```python
from build123d import *

# Parameters (mm, degrees)
F0_R     = 42
F0_R_2   = 1.5
F1_DEPTH = 5
F2_R     = 2.49999
F3_SIZE  = 2


# Not quite as in the source:
# - a fillet or chamfer is up to 0.001 mm smaller than in the source, because OpenCascade refuses the exact size


with BuildPart() as f1:
    # F0 (on Top) → F1 (new body)
    with BuildSketch(Plane.XY):
        Circle(F0_R)
        with BuildLine():
            ThreePointArc((34.3681841493, 13.6144476452), (33.928844321, 12.5537874734), (32.8681841493, 12.1144476452))
            Line((32.8681841493, 12.1144476452), (32.8681841493, -12.1144476452))
            ThreePointArc((32.8681841493, -12.1144476452), (33.928844321, -12.5537874734), (34.3681841493, -13.6144476452))
            ThreePointArc((34.3681841493, -13.6144476452), (33.4422092978, -15.000266944), (31.8075239775, -14.675107817))
            Line((31.8075239775, -14.675107817), (14.675107817, -31.8075239775))
            ThreePointArc((14.675107817, -31.8075239775), (15.000266944, -32.2941590007), (15.1144476452, -32.8681841493))
            ThreePointArc((15.1144476452, -32.8681841493), (13.6144476452, -34.3681841493), (12.1144476452, -32.8681841493))
            Line((12.1144476452, -32.8681841493), (-12.1144476452, -32.8681841493))
            ThreePointArc((-12.1144476452, -32.8681841493), (-14.1884727937, -34.254003448), (-14.675107817, -31.8075239775))
            Line((-14.675107817, -31.8075239775), (-31.8075239775, -14.675107817))
            ThreePointArc((-31.8075239775, -14.675107817), (-34.254003448, -14.1884727937), (-32.8681841493, -12.1144476452))
            Line((-32.8681841493, -12.1144476452), (-32.8681841493, 12.1144476452))
            ThreePointArc((-32.8681841493, 12.1144476452), (-34.254003448, 14.1884727937), (-31.8075239775, 14.675107817))
            Line((-31.8075239775, 14.675107817), (-14.675107817, 31.8075239775))
            ThreePointArc((-14.675107817, 31.8075239775), (-14.1884727937, 34.254003448), (-12.1144476452, 32.8681841493))
            Line((-12.1144476452, 32.8681841493), (12.1144476452, 32.8681841493))
            ThreePointArc((12.1144476452, 32.8681841493), (13.6144476452, 34.3681841493), (15.1144476452, 32.8681841493))
            ThreePointArc((15.1144476452, 32.8681841493), (15.000266944, 32.2941590007), (14.675107817, 31.8075239775))
            Line((14.675107817, 31.8075239775), (31.8075239775, 14.675107817))
            ThreePointArc((31.8075239775, 14.675107817), (33.4422092978, 15.000266944), (34.3681841493, 13.6144476452))
        make_face(mode=Mode.SUBTRACT)
        with BuildLine():
            Line((32.8681841493, -12.1144476452), (32.8681841493, 12.1144476452))
            ThreePointArc((32.8681841493, 12.1144476452), (31.4823648505, 13.0404224967), (31.8075239775, 14.675107817))
            Line((31.8075239775, 14.675107817), (14.675107817, 31.8075239775))
            ThreePointArc((14.675107817, 31.8075239775), (13.0404224967, 31.4823648505), (12.1144476452, 32.8681841493))
            Line((12.1144476452, 32.8681841493), (-12.1144476452, 32.8681841493))
            ThreePointArc((-12.1144476452, 32.8681841493), (-13.0404224967, 31.4823648505), (-14.675107817, 31.8075239775))
            Line((-14.675107817, 31.8075239775), (-31.8075239775, 14.675107817))
            ThreePointArc((-31.8075239775, 14.675107817), (-31.4823648505, 14.1884727937), (-31.3681841493, 13.6144476452))
            ThreePointArc((-31.3681841493, 13.6144476452), (-31.8075239775, 12.5537874734), (-32.8681841493, 12.1144476452))
            Line((-32.8681841493, 12.1144476452), (-32.8681841493, -12.1144476452))
            ThreePointArc((-32.8681841493, -12.1144476452), (-31.8075239775, -12.5537874734), (-31.3681841493, -13.6144476452))
            ThreePointArc((-31.3681841493, -13.6144476452), (-31.4823648505, -14.1884727937), (-31.8075239775, -14.675107817))
            Line((-31.8075239775, -14.675107817), (-14.675107817, -31.8075239775))
            ThreePointArc((-14.675107817, -31.8075239775), (-13.0404224967, -31.4823648505), (-12.1144476452, -32.8681841493))
            Line((-12.1144476452, -32.8681841493), (12.1144476452, -32.8681841493))
            ThreePointArc((12.1144476452, -32.8681841493), (13.0404224967, -31.4823648505), (14.675107817, -31.8075239775))
            Line((14.675107817, -31.8075239775), (31.8075239775, -14.675107817))
            ThreePointArc((31.8075239775, -14.675107817), (31.4823648505, -13.0404224967), (32.8681841493, -12.1144476452))
        make_face()
        with Locations((-5, -5)):
            Circle(F0_R_2, mode=Mode.SUBTRACT)
        with Locations((5, -5)):
            Circle(F0_R_2, mode=Mode.SUBTRACT)
        with Locations((-5, 5)):
            Circle(F0_R_2, mode=Mode.SUBTRACT)
        with Locations((5, 5)):
            Circle(F0_R_2, mode=Mode.SUBTRACT)
    extrude(amount=F1_DEPTH)

    # F2 (radius 2.5 in the source; OpenCascade refuses exactly that, so slightly less here)
    f2_edges = [f1.edges().sort_by_distance(p)[0] for p in [
        (42, 0, 2.5),
        (-42, 0, 0),
        (-42, 0, 5),
    ]]
    fillet(f2_edges, radius=F2_R)

    # F3
    f3_edges = [f1.edges().sort_by_distance(p)[0] for p in [
        (-34.368184, 13.614448, 5),
        (-12.553787, 33.928844, 5),
        (15.114448, 32.868184, 5),
        (33.928844, 12.553787, 5),
        (32.868184, -15.114448, 5),
        (-15.114448, -32.868184, 5),
        (12.553787, -33.928844, 5),
        (-34.368184, -13.614448, 5),
        (-6.5, -5, 0),
        (-6.5, 5, 0),
        (3.5, 5, 0),
        (3.5, -5, 0),
    ]]
    chamfer(f3_edges, length=F3_SIZE)


solid = f1.part
```
For this review, take the finished solid that the model builds, in its own axes (mm). Round coordinates to 2 decimals unless told otherwise and drop trailing zeros. Put each result on its own line as item: value.
Q1. Mouldability with a two-part tool opening along Y and no side actions: class faces 1 (the face through (-1, 1, 5)), 2 (the face through (-6.2, 4.1, 3.5)) as released by +Y, released by -Y, zero draft, split by the parting line, or undercut.
Solved:
face 1: zero draft
face 2: undercut
Q2. Wall thickness on probe 1 along X at (y, z) = (-34, 3.35); probe 2 along Y at (x, z) = (5, 2.9); probe 3 along X at (y, z) = (34.5, 4.15): over which ranges is each line inside the solid? List them lowest first.
Solved:
probe 1: x = -24.4 to -15.08, -12.15 to 12.15, 15.08 to 24.4
probe 2: y = -41.67 to -6.5, -3.5 to 3.5, 6.5 to 41.67
probe 3: x = -22.85 to -15.7, -11.53 to 11.53, 15.7 to 22.85
Q3. We need section A-A (z = 3.8). Count the separate pieces of the cut face and the enclosed holes in it, and give its area (3 significant figures).
Solved:
separate pieces: 1
enclosed holes: 12
area: 5,280 mm2
Q4. Insertion check: pin 1 Ø2 at (y, z) = (-32.5, 2) entering from -X; pin 2 Ø1 at (x, z) = (24.5, 3.5) entering from -Y; pin 3 Ø2.5 at (x, y) = (5, -5) entering from -Z; pin 4 Ø1.5 at (x, z) = (8, 1.5) entering from -Y. Each pin has a flat end and moves straight along its axis. Give the tip position at first contact, or say it passes through.
Solved:
pin 1: stops at x = -27.73
pin 2: stops at y = -34.28
pin 3: passes through
pin 4: stops at y = -41.29
